Can you work these out from the drawing? Everything is in mm from the part's minimum corner. Round coordinates to 2 decimals unless told otherwise and drop trailing zeros. One line per item, written item: value.
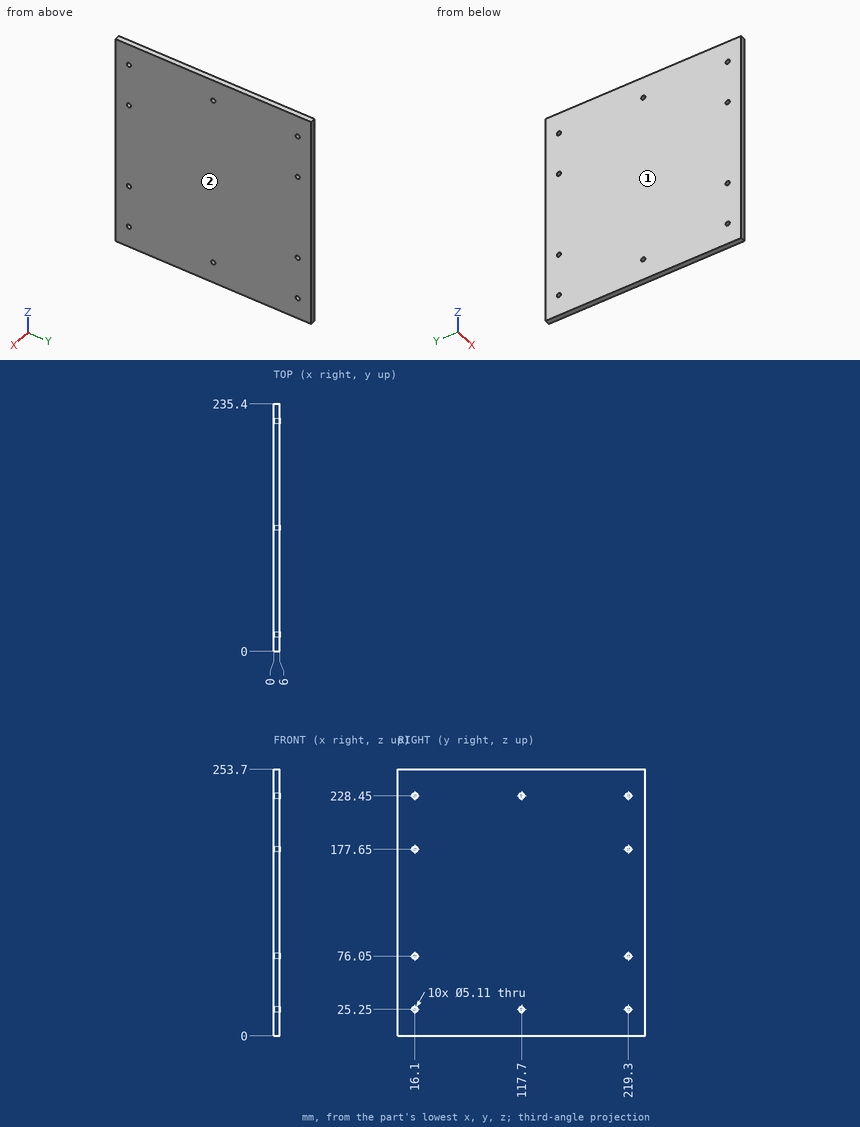
Q1. Please list where these lines run through material, in increasing order: line 1 along Z through (x, y) = (1.8, 117.7) (3 decimals); line 2 along Z through (x, y) = (3.9, 219.3) (3 decimals); line 3 along Y through (x, z) = (4.25, 76.05) (3 decimals).
Answers below:
line 1: 0 to 22.695, 27.805 to 225.895, 231.005 to 253.7
line 2: 0 to 22.695, 27.805 to 73.495, 78.605 to 175.095, 180.205 to 225.895, 231.005 to 253.7
line 3: 0 to 13.545, 18.655 to 216.745, 221.855 to 235.4
Q2. Will these pins go through, and if not, where does the flat tip stop? pin 1 Ø6 at (y, z) = (219.3, 76.05) entering from +X; pin 2 Ø4.5 at (y, z) = (117.7, 228.45) entering from -X.
Answers below:
pin 1: x = 6
pin 2: through
Q3. We'd pull the mould along X, two halves only. Please class the marked faces 1 and 2: released by +X, released by -X, zero draft, split by the parting line, or undercut.
Answers below:
face 1: released by -X
face 2: released by +X
